from build123d import *

# Parameters (mm, degrees)
F0_W     = 2.5
F0_H     = 2
F2_DEPTH = 4
F3_R     = 0.2


with BuildPart() as f1:
    # F0 (on Front) → F1 (revolve)
    with BuildSketch(Plane.XZ):
        with Locations((-1.25, 5.75)):
            Rectangle(F0_W, F0_H)
    revolve(axis=Axis((0, 0, 1), (0, 0, -1)))

    # F0 (on Front) → F2 (join, symmetric)
    with BuildSketch(Plane.XZ):
        Polygon((4, -4.75), (4, 4.75), (2.5, 4.75), (0, 4.75), (0, -4.75), align=None)
        Polygon((0, -4.75), (0, 4.75), (-2.5, 4.75), (-4, 4.75), (-4, -4.75), align=None)
    extrude(amount=F2_DEPTH, both=True)

    # F3
    f3_edges = [f1.edges().sort_by_distance(p)[0] for p in [
        (2.5, 0, 6.75),
    ]]
    fillet(f3_edges, radius=F3_R)


solid = f1.part
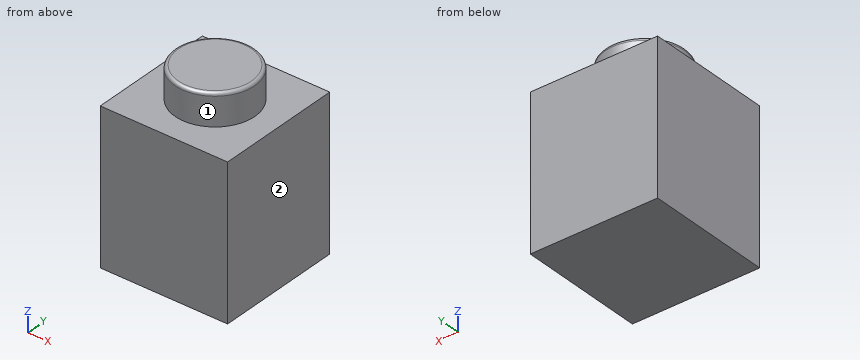
Could you check a few things on this model? Use its own coordinates, in mm. Face numbers are marked on the shaded views. A direction names the side the tool comes from. Coordinates: 2 decimals unless noted, no trailing zeros. Order: outer loops, then holes, each group sorted by start corner. A loop starts at its lowest first (then second) coordinate and runs counter-clockwise, first axis right, second up.
Q1. Please list where this line runs through material, in increasing order: L1, parallel to Z at x = 0.5, y = -2.75.
Q2. Suppose I cut it at D-D on x = 2.75. Please give me the cut outline in (y, z).
Q3. Suppose I cut it at C-C on z = 6. Please give me the cut outline in (x, y), and give its area (3 significant figures).
Q4. Suppose I cut it at A-A on y = 0. Please give me the cut outline in (x, z).
Q5. Which directions (+Z, -Z, +X, -X, +Y, -Y) give clear straight access to the entire face, cutting with the end or side of a thin tool? Please do the marked faces 1 and 2.
Answer:
1. L1: z = -4.75 to 4.75
2. outline: (-4, -4.75) - (4, -4.75) - (4, 4.75) - (-4, 4.75) - close
3. outline: circle Ø5 at (0, 0)
3. area: 19.6 mm2
4. outline: (-4, -4.75) - (4, -4.75) - (4, 4.75) - (2.5, 4.75) - (2.5, 6.55) arc R0.2 ccw to (2.3, 6.75) - (-2.3, 6.75) arc R0.2 ccw to (-2.5, 6.55) - (-2.5, 4.75) - (-4, 4.75) - close
5. face 1: +Z
5. face 2: +Z, -Z, +X, +Y, -Y
